Read the model definition and answer for the solid it produces. Units are mm, in the model's axes. Coordinates: 2 decimals unless noted, no trailing zeros. Loops run counter-clockwise (first coordinate to the right, second up) from the corner with the lowest first, then second, coordinate; pieces in that order, holes last. Notation, with made-up numbers: M 0.5,58 L 43.5,58 A18 ccw 43.5,88 Z; hole C -13.5,-36.75 d6. An arc over 180 degrees is marked long. One line per item, written item: value. Start each with the question number.
1. The part is cut by section C-C (x = 1.5). Write down the section's boundary in (y, z).
2. The part is cut by section B-B (z = 4.25). State how many separate pieces and enclosed holes the cut face has, then the cut area to 3 significant figures.
3. Determine the mould class of faces 1 (the face through (-3, 11, 5)), 2 (the face through (-13.98, 51.01, 2.54)), 3 (the face through (-21.15, -15.12, 2.46)) for opening direction Y: +Y half, -Y half, draft (parallel to the pull), parting line (faces both ways), or undercut.
4. Flat-ended cylindrical pins translate along their axes: pin 1 (1.5 mm diameter, centred on y = -9, z = 2.5, fed in from +X); pin 2 (1.8 mm diameter, centred on x = 10.02, y = -12.76, fed in from -Z). Find the tip coordinate at first contact, or state that the pin passes through.
5. Consider probe 1 along Y at (x, z) = (-5, 1.8); probe 2 along Y at (x, z) = (-3.5, 1); probe 3 along Y at (x, z) = (-4, 1.15). Determine where each line is inside the solid, lowest interval first.
6. The part is cut by section A-A (x = -12). Write down the section's boundary in (y, z), then the cut area to 3 significant figures.
7. The part is cut by section D-D (y = -18). Write down the section's boundary in (x, z), then the cut area to 3 significant figures.
```python
from build123d import *

# Parameters (mm, degrees)
EXTRUDE_1_DEPTH     = 5
SKETCH_2_R          = 5
CUT_EXTRUDE_1_DEPTH = 5
CUT_EXTRUDE_2_REACH = 75.385
SKETCH_3_R          = 1.5


with BuildPart() as part:
    # 草图1 → 凸台-拉伸1 (new body)
    with BuildSketch(Plane.XY):
        with BuildLine():
            Line((-22.282205337, 49.741076161), (-22.282205337, -5.258923839))
            Line((-22.282205337, -5.258923839), (-19.982205337, -25.258923839))
            Line((-19.982205337, -25.258923839), (-14.482205337, -50.258923839))
            Line((-14.482205337, -50.258923839), (-9.482205337, -50.258923839))
            Line((-9.482205337, -50.258923839), (10.517794663, -25.258923839))
            Line((10.517794663, -25.258923839), (17.717794663, -5.258923839))
            Line((17.717794663, -5.258923839), (17.717794663, 49.741076161))
            ThreePointArc((17.717794663, 49.741076161), (-2.282205337, 69.741076161), (-22.282205337, 49.741076161))
        make_face()
    extrude(amount=EXTRUDE_1_DEPTH)

    # 草图2 → 切除-拉伸1 (cut)
    with BuildSketch(Plane.XY.offset(5)):
        with Locations((-2.282205337, 49.741076161)):
            Circle(SKETCH_2_R)
    extrude(amount=-CUT_EXTRUDE_1_DEPTH, mode=Mode.SUBTRACT)

    # 草图3 → 切除-拉伸2 (cut, up to next)
    with BuildSketch(Plane.XY.offset(5), mode=Mode.PRIVATE) as cut_extrude_2_sk1:
        with Locations((-11.982205337, -37.758923839)):
            Circle(SKETCH_3_R)
    cut_extrude_2_tool1 = extrude(cut_extrude_2_sk1.sketch, amount=-CUT_EXTRUDE_2_REACH, mode=Mode.PRIVATE) & part.part
    # 草图3 → 切除-拉伸2 (cut, up to next)
    with BuildSketch(Plane.XY.offset(5), mode=Mode.PRIVATE) as cut_extrude_2_sk2:
        with Locations((-14.782205337, 49.741076161)):
            Circle(SKETCH_3_R)
    cut_extrude_2_tool2 = extrude(cut_extrude_2_sk2.sketch, amount=-CUT_EXTRUDE_2_REACH, mode=Mode.PRIVATE) & part.part
    # 草图3 → 切除-拉伸2 (cut, up to next)
    with BuildSketch(Plane.XY.offset(5), mode=Mode.PRIVATE) as cut_extrude_2_sk3:
        with Locations((10.217794663, 49.741076161)):
            Circle(SKETCH_3_R)
    cut_extrude_2_tool3 = extrude(cut_extrude_2_sk3.sketch, amount=-CUT_EXTRUDE_2_REACH, mode=Mode.PRIVATE) & part.part
    # 草图3 → 切除-拉伸2 (cut, up to next)
    with BuildSketch(Plane.XY.offset(5), mode=Mode.PRIVATE) as cut_extrude_2_sk4:
        with Locations((-2.282205337, 62.241076161)):
            Circle(SKETCH_3_R)
    cut_extrude_2_tool4 = extrude(cut_extrude_2_sk4.sketch, amount=-CUT_EXTRUDE_2_REACH, mode=Mode.PRIVATE) & part.part
    # 草图3 → 切除-拉伸2 (cut, up to next)
    with BuildSketch(Plane.XY.offset(5), mode=Mode.PRIVATE) as cut_extrude_2_sk5:
        with Locations((10.217794663, 22.241076161)):
            Circle(SKETCH_3_R)
    cut_extrude_2_tool5 = extrude(cut_extrude_2_sk5.sketch, amount=-CUT_EXTRUDE_2_REACH, mode=Mode.PRIVATE) & part.part
    # 草图3 → 切除-拉伸2 (cut, up to next)
    with BuildSketch(Plane.XY.offset(5), mode=Mode.PRIVATE) as cut_extrude_2_sk6:
        with Locations((-14.782205337, 22.241076161)):
            Circle(SKETCH_3_R)
    cut_extrude_2_tool6 = extrude(cut_extrude_2_sk6.sketch, amount=-CUT_EXTRUDE_2_REACH, mode=Mode.PRIVATE) & part.part
    # 草图3 → 切除-拉伸2 (cut, up to next)
    with BuildSketch(Plane.XY.offset(5), mode=Mode.PRIVATE) as cut_extrude_2_sk7:
        with Locations((-16.419705337, -12.758923839)):
            Circle(SKETCH_3_R)
    cut_extrude_2_tool7 = extrude(cut_extrude_2_sk7.sketch, amount=-CUT_EXTRUDE_2_REACH, mode=Mode.PRIVATE) & part.part
    # 草图3 → 切除-拉伸2 (cut, up to next)
    with BuildSketch(Plane.XY.offset(5), mode=Mode.PRIVATE) as cut_extrude_2_sk8:
        with Locations((10.017794663, -12.758923839)):
            Circle(SKETCH_3_R)
    cut_extrude_2_tool8 = extrude(cut_extrude_2_sk8.sketch, amount=-CUT_EXTRUDE_2_REACH, mode=Mode.PRIVATE) & part.part
    add(cut_extrude_2_tool1.solids().sort_by_distance((-11.982205, -37.758924, 5))[0], mode=Mode.SUBTRACT)
    add(cut_extrude_2_tool2.solids().sort_by_distance((-14.782205, 49.741076, 5))[0], mode=Mode.SUBTRACT)
    add(cut_extrude_2_tool3.solids().sort_by_distance((10.217795, 49.741076, 5))[0], mode=Mode.SUBTRACT)
    add(cut_extrude_2_tool4.solids().sort_by_distance((-2.282205, 62.241076, 5))[0], mode=Mode.SUBTRACT)
    add(cut_extrude_2_tool5.solids().sort_by_distance((10.217795, 22.241076, 5))[0], mode=Mode.SUBTRACT)
    add(cut_extrude_2_tool6.solids().sort_by_distance((-14.782205, 22.241076, 5))[0], mode=Mode.SUBTRACT)
    add(cut_extrude_2_tool7.solids().sort_by_distance((-16.419705, -12.758924, 5))[0], mode=Mode.SUBTRACT)
    add(cut_extrude_2_tool8.solids().sort_by_distance((10.017795, -12.758924, 5))[0], mode=Mode.SUBTRACT)


solid = part.part
```
Answer block:
1. outline: M -36.53,0 L 46.47,0 L 46.47,5 L -36.53,5 Z; M 53.01,0 L 69.38,0 L 69.38,5 L 53.01,5 Z
2. separate pieces: 1
2. enclosed holes: 9
2. area: 3,840 mm2
3. face 1: draft
3. face 2: undercut
3. face 3: -Y half
4. pin 1: stops at x = 16.64
4. pin 2: passes through
5. probe 1: y = -44.66 to 45.54, 53.94 to 69.56
5. probe 2: y = -42.78 to 44.89, 54.59 to 61.37, 63.12 to 69.7
5. probe 3: y = -43.41 to 45.05, 54.44 to 69.67
6. outline: M -50.26,0 L -39.26,0 L -39.26,5 L -50.26,5 Z; M -36.26,0 L 67.22,0 L 67.22,5 L -36.26,5 Z
6. area: 572 mm2
7. outline: M -20.82,0 L 13.13,0 L 13.13,5 L -20.82,5 Z
7. area: 170 mm2
